Read the model definition and answer for the solid it produces. Units are mm, in the model's axes. Face numbers are marked on the shaded views. A direction names the side the tool comes from. Coordinates: 2 decimals unless noted, no trailing zeros. Order: outer loops, then holes, each group sorted by start corner. A loop starts at its lowest first (then second) coordinate and runs counter-clockwise, first axis right, second up. Notation, with made-up numbers: (84, 66) -> (134, 66) arc R25 cw to (134, 89) -> close; hole circle Ø5 at (-33, 20.5). An arc over 180 degrees is marked (long way). Answer as a JSON object with one key per item and string values. Group by question number.
1) Section C-C on y = -23.1 is taken. Determine the outline of the cut face in (x, z).
2) Section B-B on z = 16.5 is taken. Count the separate pieces of the cut face and the enclosed holes in it, and give its area (3 significant figures).
3) Given pin 1 (1.3 mm diameter, centred on y = 36, z = 7, fed in from +X); pin 2 (4 mm diameter, centred on y = -18.5, z = 11.5, fed in from +X); pin 3 (2 mm diameter, centred on x = -8, z = 15, fed in from +Y); pin 4 (1 mm diameter, centred on y = -3, z = 12.5, fed in from -X), each flat-ended and moving along its own axis, determine where each tip first touches the part or whether it passes through.
4) Consider L1, parallel to Y at x = -22, z = 11; L2, parallel to Y at x = 13.4, z = 2.05; L3, parallel to X at y = -12, z = 5. Determine where each line is inside the solid, lowest interval first.
5) Section A-A on x = 13.4 is taken. Determine the outline of the cut face in (y, z), and give its area (3 significant figures).
6) A tool of negligible diameter and unlimited length cuts with its end or side. For the marked faces 4, 5 and 6, from which of +Z, -Z, +X, -X, +Y, -Y can it reach the whole face along a straight path? Write none if from no direction.
7) Section D-D on x = 0.5 is taken. Determine the outline of the cut face in (y, z), and give its area (3 significant figures).
8) Determine the mould class of the marked faces 1, 2 and 3 for opening direction X: released by +X, released by -X, zero draft, split by the parting line, or undercut.
from build123d import *

# Parameters (mm, degrees)
CROQUIS1_W              = 50.8
CROQUIS1_H              = 76.2
SALIENTE_EXTRUIR1_DEPTH = 18
CROQUIS2_W              = 50.8
CROQUIS2_H              = 76.2
CROQUIS2_W_2            = 46.12
CROQUIS2_H_2            = 71.52
CROQUIS2_W_3            = 38.8
CROQUIS2_H_3            = 64.2
CORTAR_EXTRUIR1_DEPTH   = 15
CORTAR_EXTRUIR8_DEPTH   = 15
SALIENTE_EXTRUIR3_DEPTH = 41.5
CORTAR_EXTRUIR9_DEPTH   = 51.5
CORTAR_EXTRUIR10_DEPTH  = 51.5
SALIENTE_EXTRUIR4_DEPTH = 16
CORTAR_EXTRUIR11_DEPTH  = 16.5
REDONDEO3_R             = 2
REDONDEO4_R             = 1
CROQUIS15_W             = 48.12
CROQUIS15_H             = 10
CORTAR_EXTRUIR12_DEPTH  = 15
CROQUIS16_W             = 8
CROQUIS16_H             = 1.5
CORTAR_EXTRUIR13_DEPTH  = 2
CROQUIS17_R             = 3
CORTAR_EXTRUIR14_DEPTH  = 10


with BuildPart() as part:
    # Croquis1 → Saliente-Extruir1 (new body)
    with BuildSketch(Plane.XY):
        Rectangle(CROQUIS1_W, CROQUIS1_H)
    extrude(amount=SALIENTE_EXTRUIR1_DEPTH)

    # Croquis2 → Cortar-Extruir1 (cut)
    # profile 1 of 2: a face of its own
    with BuildSketch(Plane.XY.offset(18)):
        Rectangle(CROQUIS2_W, CROQUIS2_H)
        Rectangle(CROQUIS2_W_2, CROQUIS2_H_2, mode=Mode.SUBTRACT)
    # profile 2 of 2: a face of its own
    with BuildSketch(Plane.XY.offset(18)):
        Rectangle(CROQUIS2_W_3, CROQUIS2_H_3)
    extrude(amount=-CORTAR_EXTRUIR1_DEPTH, mode=Mode.SUBTRACT)

    # Croquis6 → Cortar-Extruir8 (cut)
    with BuildSketch(Plane.XY.offset(18)):
        Polygon((-23.06, 35.76), (-8.06, 35.76), (-8.06, 32.1), (-19.4, 32.1), (-19.4, 20.76), (-23.06, 20.76), align=None)
        Polygon((23.06, 35.76), (8.06, 35.76), (8.06, 32.1), (19.4, 32.1), (19.4, 20.76), (23.06, 20.76), align=None)
        Polygon((-23.06, -35.76), (-23.06, -20.76), (-19.4, -20.76), (-19.4, -32.1), (-8.06, -32.1), (-8.06, -35.76), align=None)
        Polygon((23.06, -35.76), (8.06, -35.76), (8.06, -32.1), (19.4, -32.1), (19.4, -20.76), (23.06, -20.76), align=None)
    extrude(amount=-CORTAR_EXTRUIR8_DEPTH, mode=Mode.SUBTRACT)

    # Croquis10 → Saliente-Extruir3 (add)
    with BuildSketch(Plane(origin=(0, -20.76, 0), x_dir=(-1, 0, 0), z_dir=(0, -1, 0))):
        Polygon((23.06, -18), (24.06, -18), (23.06, -3), align=None)
        Polygon((-23.06, -18), (-24.06, -18), (-23.06, -3), align=None)
    extrude(amount=-SALIENTE_EXTRUIR3_DEPTH)

    # Croquis11 → Cortar-Extruir9 (cut)
    with BuildSketch(Plane.XZ.offset(20.76)):
        Polygon((-19.4, 18), (-21.56, 18), (-20.56, 3), (-19.4, 3), align=None)
    extrude(amount=-CORTAR_EXTRUIR9_DEPTH, mode=Mode.SUBTRACT)

    # Croquis12 → Cortar-Extruir10 (cut)
    with BuildSketch(Plane.XZ.offset(20.76)):
        Polygon((19.4, 18), (19.4, 3), (20.56, 3), (21.56, 18), align=None)
    extrude(amount=-CORTAR_EXTRUIR10_DEPTH, mode=Mode.SUBTRACT)

    # Croquis13 → Saliente-Extruir4 (add)
    with BuildSketch(Plane(origin=(8.06, 0, 0), x_dir=(0, 0, -1), z_dir=(1, 0, 0))):
        Polygon((-18, -35.76), (-18, -37.76), (-3, -35.76), align=None)
        Polygon((-18, 35.76), (-18, 37.76), (-3, 35.76), align=None)
    extrude(amount=-SALIENTE_EXTRUIR4_DEPTH)

    # Croquis14 → Cortar-Extruir11 (cut)
    with BuildSketch(Plane(origin=(8.06, 0, 0), x_dir=(0, 0, -1), z_dir=(1, 0, 0))):
        Polygon((-3, -32.1), (-18, -32.1), (-18, -35.26), (-3, -33.26), align=None)
        Polygon((-18, 32.1), (-18, 35.26), (-3, 33.26), (-3, 32.1), align=None)
    extrude(amount=-CORTAR_EXTRUIR11_DEPTH, mode=Mode.SUBTRACT)

    # Redondeo3
    redondeo3_edges = [part.edges().sort_by_distance(p)[0] for p in [
        (-25.4, 38.1, 1.5),
        (25.4, 38.1, 1.5),
        (25.4, -38.1, 1.5),
        (-25.4, -38.1, 1.5),
    ]]
    fillet(redondeo3_edges, radius=REDONDEO3_R)

    # Redondeo4
    redondeo4_edges = [part.edges().sort_by_distance(p)[0] for p in [
        (0, 38.1, 0),
        (-25.4, 0, 0),
        (25.4, 0, 0),
        (0, -38.1, 0),
        (24.814213562, -37.514213562, 0),
        (-24.814213562, -37.514213562, 0),
        (-24.814213562, 37.514213562, 0),
        (24.814213562, 37.514213562, 0),
    ]]
    fillet(redondeo4_edges, radius=REDONDEO4_R)

    # Croquis15 → Cortar-Extruir12 (cut)
    with BuildSketch(Plane.XY.offset(18)):
        with Locations((0, -0.01)):
            Rectangle(CROQUIS15_W, CROQUIS15_H)
    extrude(amount=-CORTAR_EXTRUIR12_DEPTH, mode=Mode.SUBTRACT)

    # Croquis16 → Cortar-Extruir13 (cut)
    with BuildSketch(Plane.XZ.offset(38.1)):
        with Locations((0, 2.25)):
            Rectangle(CROQUIS16_W, CROQUIS16_H)
    extrude(amount=-CORTAR_EXTRUIR13_DEPTH, mode=Mode.SUBTRACT)

    # Croquis17 → Cortar-Extruir14 (cut)
    with BuildSketch(Plane.XY.offset(3)):
        with Locations((13.4, -23.1)):
            Circle(CROQUIS17_R)
    extrude(amount=-CORTAR_EXTRUIR14_DEPTH, mode=Mode.SUBTRACT)


solid = part.part
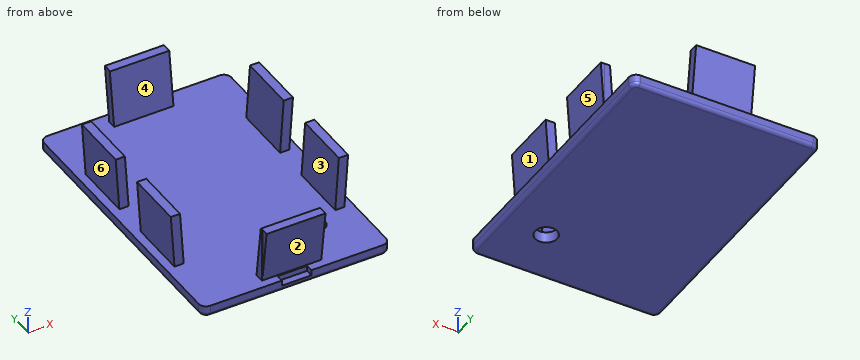
Worked answers:
{
 "1": {"outline": "(-25.4, 1) arc R1 ccw to (-24.4, 0) -> (10.4, 0) -> (10.4, 3) -> (-25.4, 3) -> close; (16.4, 0) -> (24.4, 0) arc R1 ccw to (25.4, 1) -> (25.4, 3) -> (16.4, 3) -> close"},
 "2": {"separate pieces": "6", "enclosed holes": "0", "area": "238 mm²"},
 "3": {"pin 1": "stops at x = 8.06", "pin 2": "stops at x = 23.76", "pin 3": "stops at y = 37.49", "pin 4": "passes through"},
 "4": {"L1": "y = -20.76 to -5.01, 4.99 to 20.76", "L2": "y = -38.1 to -26.1, -20.1 to 38.1", "L3": "x = -23.19 to -20.69, 20.69 to 23.19"},
 "5": {"outline": "(-38.1, 1) arc R1 ccw to (-37.1, 0) -> (-26.1, 0) -> (-26.1, 3) -> (-38.1, 3) -> close; (-20.1, 0) -> (37.1, 0) arc R1 ccw to (38.1, 1) -> (38.1, 3) -> (-20.1, 3) -> close", "area": "210 mm²"},
 "6": {"face 4": "+Z, +X, -X", "face 5": "+X, +Y, -Y", "face 6": "-X, +Y, -Y"},
 "7": {"outline": "(-38.1, 1) arc R1 ccw to (-37.1, 0) -> (37.1, 0) arc R1 ccw to (38.1, 1) -> (38.1, 3) -> (35.76, 3) -> (37.76, 18) -> (35.26, 18) -> (33.26, 3) -> (-33.26, 3) -> (-35.26, 18) -> (-37.76, 18) -> (-35.76, 3) -> (-36.1, 3) -> (-36.1, 1.5) -> (-38.1, 1.5) -> close", "area": "300 mm²"},
 "8": {"face 1": "released by +X", "face 2": "zero draft", "face 3": "undercut"}
}
